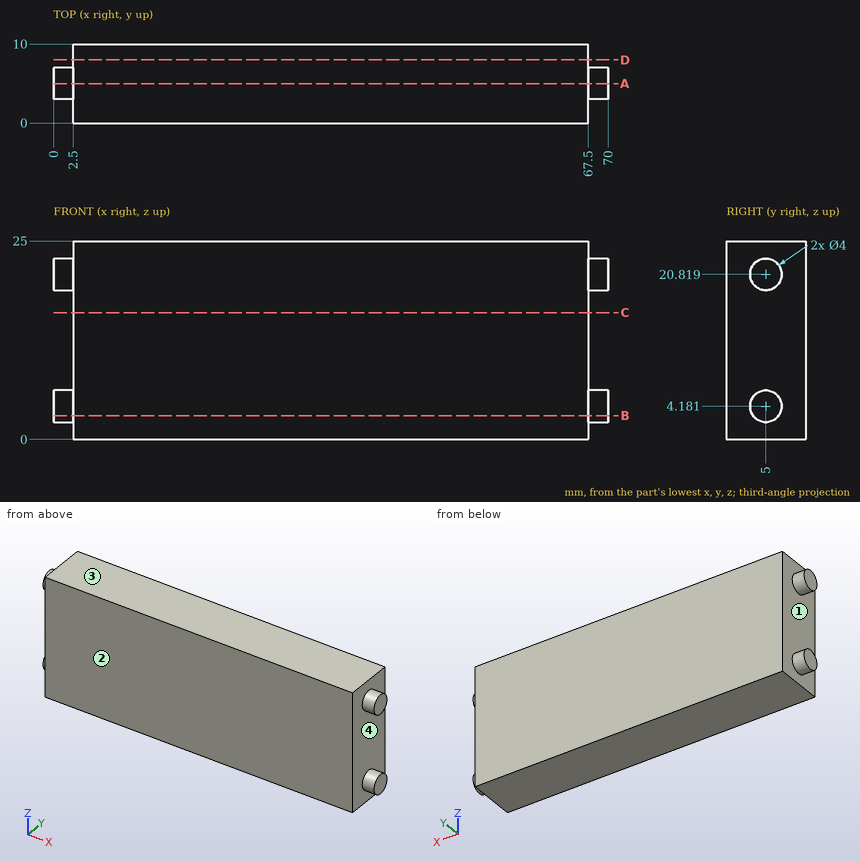
Here's the drawing with two shaded views (mm, measured from the low corner). I have some questions. Round coordinates to 2 decimals unless told otherwise and drop trailing zeros. Loops run counter-clockwise (first coordinate to the right, second up) from the corner with the lowest first, then second, coordinate; pieces in that order, holes last.
1. Suppose I cut it at B-B, the plane z = 3. Please give me the cut outline in (x, y), and give its area (3 significant figures).
Answers:
outline: (0, 3.39) - (2.5, 3.39) - (2.5, 0) - (67.5, 0) - (67.5, 3.39) - (70, 3.39) - (70, 6.61) - (67.5, 6.61) - (67.5, 10) - (2.5, 10) - (2.5, 6.61) - (0, 6.61) - close
area: 666 mm2
2. Suppose I cut it at A-A, the plane y = 5. Please give me the cut outline in (x, z), and give its area (4 significant figures).
Answers:
outline: (0, 2.18) - (2.5, 2.18) - (2.5, 0) - (67.5, 0) - (67.5, 2.18) - (70, 2.18) - (70, 6.18) - (67.5, 6.18) - (67.5, 18.82) - (70, 18.82) - (70, 22.82) - (67.5, 22.82) - (67.5, 25) - (2.5, 25) - (2.5, 22.82) - (0, 22.82) - (0, 18.82) - (2.5, 18.82) - (2.5, 6.18) - (0, 6.18) - close
area: 1,665 mm2
3. Suppose I cut it at D-D, the plane y = 8. Please give me the cut outline in (x, z).
Answers:
outline: (2.5, 0) - (67.5, 0) - (67.5, 25) - (2.5, 25) - close
4. If I drill on probe 1 along X at (y, z) = (1.5, 19.75), over which ranges is the centre line in solid material (lowest first)?
Answers:
probe 1: x = 2.5 to 67.5
5. Suppose I cut it at C-C, the plane z = 16. Please give me the cut outline in (x, y), and give its area (3 significant figures).
Answers:
outline: (2.5, 0) - (67.5, 0) - (67.5, 10) - (2.5, 10) - close
area: 650 mm2
6. Thinking about a two-plate mould opening in Z: for the marked faces 1, 2, 3 and 4, which applies, released by +Z, released by -Z, zero draft, split by the parting line, or undercut?
Answers:
face 1: undercut
face 2: zero draft
face 3: released by +Z
face 4: undercut
